```python
from build123d import *

# Parameters (mm, degrees)
BOX001_W     = 3
BOX001_H     = 4
BOX001_DEPTH = 15
BOX_W        = 3
BOX_H        = 4
BOX_DEPTH    = 15
SKETCH_W     = 200
SKETCH_H     = 90
SKETCH_R     = 1.549855
SKETCH_R_2   = 1.534707
SKETCH_R_3   = 1.450363
SKETCH_R_4   = 1.487036
SKETCH_R_5   = 1.500003
SKETCH_R_6   = 1.546382
SKETCH_R_7   = 1.475806
SKETCH_R_8   = 1.470873
SKETCH_R_9   = 1.517779
SKETCH_R_10  = 1.459473
SKETCH_R_11  = 1.474048
SKETCH_R_12  = 1.452864
SKETCH_R_13  = 1.50738
SKETCH_R_14  = 1.532562
SKETCH_R_15  = 4.638624
SKETCH_R_16  = 3
SKETCH_R_17  = 1.469531
SKETCH_R_18  = 1.503215
SKETCH_R_19  = 1.49249
SKETCH_R_20  = 1.53474
SKETCH_R_21  = 6
SKETCH_W_2   = 61
SKETCH_H_2   = 14
SKETCH_W_3   = 14
PAD_DEPTH    = 1


with BuildPart() as cube001:
    # Box001 → Box001 (new body)
    with BuildSketch(Plane(origin=(173.5, 26, -7), x_dir=(1, 0, 0), z_dir=(0, 0, 1))):
        with Locations((1.5, 2)):
            Rectangle(BOX001_W, BOX001_H)
    extrude(amount=BOX001_DEPTH)


with BuildPart() as cube:
    # Box → Box (new body)
    with BuildSketch(Plane(origin=(23.5, 25, -7), x_dir=(1, 0, 0), z_dir=(0, 0, 1))):
        with Locations((1.5, 2)):
            Rectangle(BOX_W, BOX_H)
    extrude(amount=BOX_DEPTH)


with BuildPart() as cut001:
    # Sketch → Pad (new body)
    with BuildSketch(Plane.XY):
        with Locations((100, 45)):
            Rectangle(SKETCH_W, SKETCH_H)
        with Locations((9, 82)):
            Circle(SKETCH_R, mode=Mode.SUBTRACT)
        with Locations((128, 82)):
            Circle(SKETCH_R_2, mode=Mode.SUBTRACT)
        with Locations((9, 42)):
            Circle(SKETCH_R_3, mode=Mode.SUBTRACT)
        with Locations((128, 42)):
            Circle(SKETCH_R_4, mode=Mode.SUBTRACT)
        with Locations((74, 82)):
            Circle(SKETCH_R_5, mode=Mode.SUBTRACT)
        with Locations((193, 82)):
            Circle(SKETCH_R_6, mode=Mode.SUBTRACT)
        with Locations((74, 42)):
            Circle(SKETCH_R_7, mode=Mode.SUBTRACT)
        with Locations((193, 42)):
            Circle(SKETCH_R_8, mode=Mode.SUBTRACT)
        with Locations((4, 86)):
            Circle(SKETCH_R_9, mode=Mode.SUBTRACT)
        with Locations((196, 86)):
            Circle(SKETCH_R_10, mode=Mode.SUBTRACT)
        with Locations((196, 4)):
            Circle(SKETCH_R_11, mode=Mode.SUBTRACT)
        with Locations((4, 4)):
            Circle(SKETCH_R_12, mode=Mode.SUBTRACT)
        with Locations((100, 4)):
            Circle(SKETCH_R_13, mode=Mode.SUBTRACT)
        with Locations((100, 86)):
            Circle(SKETCH_R_14, mode=Mode.SUBTRACT)
        with Locations((25, 21)):
            Circle(SKETCH_R_15, mode=Mode.SUBTRACT)
        with Locations((55, 21)):
            Circle(SKETCH_R_16, mode=Mode.SUBTRACT)
        with Locations((63, 21)):
            Circle(SKETCH_R_17, mode=Mode.SUBTRACT)
        with Locations((47, 21)):
            Circle(SKETCH_R_18, mode=Mode.SUBTRACT)
        with Locations((145, 21)):
            Circle(SKETCH_R_16, mode=Mode.SUBTRACT)
        with Locations((153, 21)):
            Circle(SKETCH_R_19, mode=Mode.SUBTRACT)
        with Locations((137, 21)):
            Circle(SKETCH_R_20, mode=Mode.SUBTRACT)
        with Locations((175, 21)):
            Circle(SKETCH_R_21, mode=Mode.SUBTRACT)
        with Locations((40.5, 66)):
            Rectangle(SKETCH_W_2, SKETCH_H_2, mode=Mode.SUBTRACT)
        with Locations((100, 66)):
            Rectangle(SKETCH_W_3, SKETCH_H_2, mode=Mode.SUBTRACT)
        with Locations((159.5, 66)):
            Rectangle(SKETCH_W_2, SKETCH_H_2, mode=Mode.SUBTRACT)
    extrude(amount=PAD_DEPTH)

    # Cut: cut Cube
    add(cube.part, mode=Mode.SUBTRACT)

    # Cut001: cut Cube001
    add(cube001.part, mode=Mode.SUBTRACT)


solid = cut001.part
```
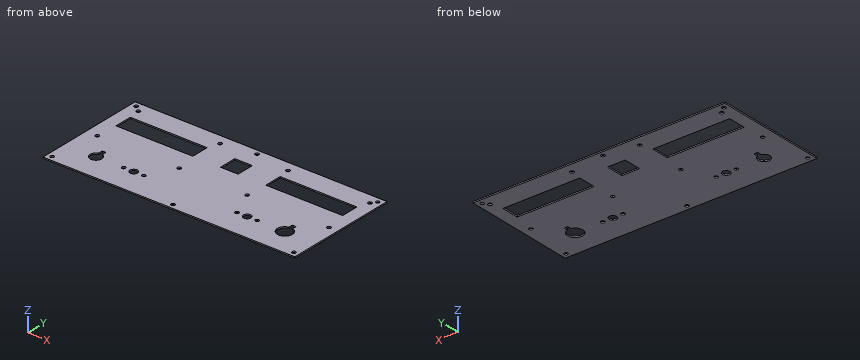
Geometry: final body of the model. Coordinates: model frame, mm. Round coordinates to 2 decimals unless told otherwise and drop trailing zeros. Write each loop counter-clockwise with the first axis right and the second up, starting at its lowest first coordinate (ties: lowest second). Pieces come first, ordered by that corner, then holes. Notation, with made-up numbers: M -1.5,61.5 L 47.5,61.5 A20 ccw 47.5,82.5 Z; hole C -6,-24.5 d10. An arc over 180 degrees is marked long. Answer in a Markdown table with one row per item. Add a question column.
(1) Ray query, L1, parallel to Y at x = 63, z = 0.35; L2, parallel to X at y = 82, z = 0.6; L3, parallel to Y at x = 4, z = 0.75. Return the intervals inside material, ascending.
(2) Cut plane B-B, the plane y = 67. Return the cut outline in (x, z).
(3) Cut plane C-C, the plane z = 0.8. Give the number of separate pieces and of enclosed holes in the cut face, then the cut area to 3 significant figures.
(4) Cut plane A-A, the plane x = 145. Return the cut outline in (y, z), then the cut area to 3 significant figures.
Established:
| question | item | result |
|---|---|---|
| 1 | L1 | 0 to 19.53, 22.47 to 59, 73 to 90 |
| 1 | L2 | 0 to 7.45, 10.55 to 72.5, 75.5 to 126.47, 129.53 to 191.45, 194.55 to 200 |
| 1 | L3 | 0 to 2.55, 5.45 to 84.48, 87.52 to 90 |
| 2 | outline | M 0,0 L 10,0 L 10,1 L 0,1 Z; M 71,0 L 93,0 L 93,1 L 71,1 Z; M 107,0 L 129,0 L 129,1 L 107,1 Z; M 190,0 L 200,0 L 200,1 L 190,1 Z |
| 3 | separate pieces | 1 |
| 3 | enclosed holes | 25 |
| 3 | area | 15,700 mm² |
| 4 | outline | M 0,0 L 18,0 L 18,1 L 0,1 Z; M 24,0 L 59,0 L 59,1 L 24,1 Z; M 73,0 L 90,0 L 90,1 L 73,1 Z |
| 4 | area | 70.0 mm² |
